Source: three-view drawing plus pictorial views. Frame: mm from the lowest corner of the part. A direction names the side the tool comes from. Give positions to 0.01 mm unless a question says otherwise; leave off trailing zeros. Loops run counter-clockwise (first coordinate to the right, second up) from the corner with the lowest first, then second, coordinate; pieces in that order, holes last. Notation, with made-up numbers: (7, -25.5) - (17, -25.5) arc R8 cw to (17, -15.5) - close; hole circle Ø4 at (50.5, 32.5). An arc over 180 degrees is marked (long way). Put each result on its own line as item: value.
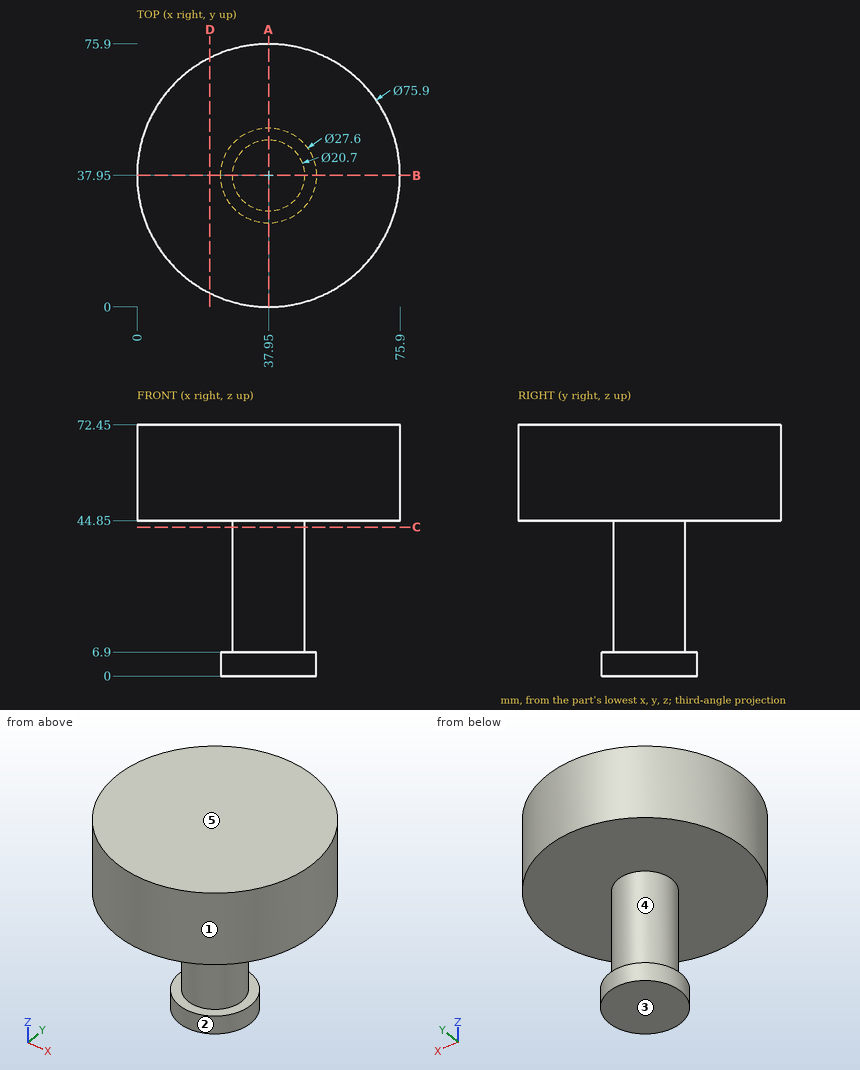
1) Pin query (flat end, axial travel): P1, Ø2, axis at y = 66, z = 60.5, coming from the +X side; P2, Ø5, axis at x = 28.5, z = 24.5, coming from the -Y side; P3, Ø6, axis at x = 21.5, z = 64, coming from the +Y side. Return the tip coordinate at first contact, or that it passes through.
Check result:
P1: x = 64.57
P2: y = 30.28
P3: y = 73.44
2) Section query C-C, the plane z = 43. Output: boundary loops of the cut face in (x, y).
Check result:
outline: circle Ø20.7 at (37.95, 37.95)
3) Access query for the marked faces 1 and 2. Directions: +Z, -Z, +X, -X, +Y, -Y. A direction counts if a zero-diameter tool reaches every point of the face in a straight line with its end or side. Return the directions, or none.
Check result:
face 1: +Z, -Z
face 2: -Z
4) Section query D-D, the plane x = 21. Output: boundary loops of the cut face in (y, z), plus the area to 3 significant figures.
Check result:
outline: (4, 44.85) - (71.9, 44.85) - (71.9, 72.45) - (4, 72.45) - close
area: 1,870 mm²
5) Material intervals for line 1 along Z through (x, y) = (43.5, 47.5); line 2 along Z through (x, y) = (45, 17.5); line 3 along Y through (x, z) = (37.5, 46.5), sorted ascending. Write a range as [from, to].
Check result:
line 1: [0, 6.9], [44.85, 72.45]
line 2: [44.85, 72.45]
line 3: [0, 75.9]
6) Mould query, pull axis Z, two halves, no side actions, for the marked faces 3, 4 and 5. Classes: pulls with the +Z half, pulls with the -Z half, needs draft (parallel to the pull), parting line crosses it, or undercut.
Check result:
face 3: pulls with the -Z half
face 4: undercut
face 5: pulls with the +Z half
7) Section query A-A, the plane x = 37.95. Output: boundary loops of the cut face in (y, z), plus the area to 3 significant figures.
Check result:
outline: (0, 44.85) - (27.6, 44.85) - (27.6, 6.9) - (24.15, 6.9) - (24.15, 0) - (51.75, 0) - (51.75, 6.9) - (48.3, 6.9) - (48.3, 44.85) - (75.9, 44.85) - (75.9, 72.45) - (0, 72.45) - close
area: 3,070 mm²
